Work out the finished part from the listing and answer in its coordinate system (mm). A direction names the side the tool comes from. Coordinates: 2 decimals unless noted, no trailing zeros. Order: outer loops, then holes, each group sorted by start corner. A loop starts at its lowest first (then second) coordinate and runs counter-clockwise, first axis right, second up. Notation, with made-up numbers: (-15, 12) -> (34, 12) arc R25 cw to (34, 48) -> close; hole circle Ø9 at (-22, 80). An arc over 180 degrees is marked (long way). Answer as CSV lines item,"result". Start each with the question number.
Item 1: Each of these flat-tipped pins is pushed along its axis until it touches: pin 1 Ø6 at (x, y) = (22, -3.5) entering from -Z; pin 2 Ø9.5 at (x, y) = (-26, -29.5) entering from -Z; pin 3 Ø8 at (x, z) = (-22.5, -22.5) entering from +Y; pin 4 Ø21 at (y, z) = (19, 26) entering from -X. Where does it stop, or does it pass through?
Item 2: Section D-D (y = 8) is taken. Write down the section's boundary in (x, z).
Item 3: Section A-A (z = 19.05) is taken. Write down the section's boundary in (x, y) (3 decimals).
Item 4: Section C-C (z = 2) is taken. Write down the section's boundary in (x, y).
Item 5: Straight lines are drawn through the part: L1, parallel to X at y = 1.85, z = 10; L2, parallel to Z at x = 5, y = 2; L3, parallel to Y at x = 34.8, z = -19.05 (3 decimals). For each, find the intervals that lie inside material, in ascending order.
Item 6: Which of the six approach directions +Z, -Z, +X, -X, +Y, -Y give full straight-line access (tool end or side, diameter ignored) to faces 1 (the face through (-5, 15, 27)), 2 (the face through (0, 15, -27)), 3 (the face through (-26, -15, -6.35))?
Item 7: Section B-B (x = 28.1) is taken. Write down the section's boundary in (y, z).
Item 8: For a pull along Y with two mould halves and no side action, classify faces 4 (the face through (5.03, 2.46, 11.5)), 5 (the face through (-29.69, -32.47, 0.09)), 6 (the face through (-2.46, 14.39, 12.36)) as pulls with the +Y half, pulls with the -Y half, needs draft (parallel to the pull), parting line crosses it, or undercut.
```python
from build123d import *

# Parameters (mm, degrees)
SKETCH2_W           = 76.2
SKETCH2_H           = 76.2
SKETCH2_R           = 1.5
BOSS_EXTRUDE1_DEPTH = 5
SKETCH3_W           = 76.2
SKETCH3_H           = 24.05
SKETCH3_R           = 4
BOSS_EXTRUDE2_DEPTH = 5
LPATTERN1_COUNT     = 2
LPATTERN1_PITCH     = 38.1
BOSS_EXTRUDE5_START = -38.1
SKETCH4_R           = 3
BOSS_EXTRUDE5_DEPTH = 6.35
CUT_EXTRUDE1_DEPTH  = 10


with BuildPart() as part:
    # Sketch2 → Boss-Extrude1 (new body)
    with BuildSketch(Plane(origin=(0, 0, 0), x_dir=(1, 0, 0), z_dir=(0, 1, 0))):
        Rectangle(SKETCH2_W, SKETCH2_H)
        with Locations(Location((28.1, 10, 0), (0, 0, 270))):
            Circle(SKETCH2_R, mode=Mode.SUBTRACT)
        with Locations(Location((5.1, 10, 0), (0, 0, 270))):
            Circle(SKETCH2_R, mode=Mode.SUBTRACT)
        with Locations(Location((28.1, -10, 0), (0, 0, 90))):
            Circle(SKETCH2_R, mode=Mode.SUBTRACT)
        with Locations(Location((5.1, -10, 0), (0, 0, 90))):
            Circle(SKETCH2_R, mode=Mode.SUBTRACT)
    extrude(amount=BOSS_EXTRUDE1_DEPTH)

    # Sketch3 → Boss-Extrude2 (add)
    with BuildSketch(Plane(origin=(38.1, 0, 0), x_dir=(0, 0, -1), z_dir=(1, 0, 0))):
        with Locations((0, 12.025)):
            Rectangle(SKETCH3_W, SKETCH3_H)
        with Locations((-19.05, 14.525)):
            Circle(SKETCH3_R, mode=Mode.SUBTRACT)
        with Locations((19.05, 14.525)):
            Circle(SKETCH3_R, mode=Mode.SUBTRACT)
    boss_extrude2 = extrude(amount=-BOSS_EXTRUDE2_DEPTH)

    # LPattern1: Boss-Extrude2 ×2
    with Locations(*[(-i * LPATTERN1_PITCH, 0, 0) for i in range(1, LPATTERN1_COUNT)]):
        add(boss_extrude2)

    # Sketch4 → Boss-Extrude5 (add, symmetric)
    with BuildSketch(Plane(origin=(0, 0, -38.1), x_dir=(-1, 0, 0), z_dir=(0, 0, -1)).offset(BOSS_EXTRUDE5_START)):
        with BuildLine():
            Line((6.1, 0), (38.1, 0))
            Line((38.1, 0), (38.1, -35.148267781))
            ThreePointArc((38.1, -35.148267781), (34.438424912, -39.965800215), (28.816552498, -37.72742995))
            Line((28.816552498, -37.72742995), (6.1, 0))
        make_face()
        with Locations((31.9, -34.5)):
            Circle(SKETCH4_R, mode=Mode.SUBTRACT)
    extrude(amount=BOSS_EXTRUDE5_DEPTH, both=True)

    # Sketch5 → Cut-Extrude1 (cut)
    with BuildSketch(Plane(origin=(0, 0, 0), x_dir=(0, 0, -1), z_dir=(1, 0, 0))):
        Polygon((9.743329583, 5), (-9.743329583, 5), (-15.05, 24.05), (-9.743329583, 24.05), (9.743329583, 24.05), (15.05, 24.05), align=None)
    extrude(amount=-CUT_EXTRUDE1_DEPTH, mode=Mode.SUBTRACT)


solid = part.part
```
Checked values:
1,pin 1,"passes through"
1,pin 2,"stops at z = -6.35"
1,pin 3,"stops at y = 5"
1,pin 4,"stops at x = -5"
2,outline,"(-5, -38.1) -> (0, -38.1) -> (0, -10.58) -> (-5, -10.58) -> close; (-5, 10.58) -> (0, 10.58) -> (0, 38.1) -> (-5, 38.1) -> close; (33.1, -38.1) -> (38.1, -38.1) -> (38.1, 38.1) -> (33.1, 38.1) -> close"
3,outline,"(-38.1, 0) -> (38.1, 0) -> (38.1, 10.525) -> (33.1, 10.525) -> (33.1, 5) -> (0, 5) -> (0, 10.525) -> (-5, 10.525) -> (-5, 5) -> (-38.1, 5) -> close; (-5, 18.525) -> (0, 18.525) -> (0, 24.05) -> (-5, 24.05) -> close; (33.1, 18.525) -> (38.1, 18.525) -> (38.1, 24.05) -> (33.1, 24.05) -> close"
4,outline,"(-38.1, -35.15) arc R5 ccw to (-28.82, -37.73) -> (-6.1, 0) -> (38.1, 0) -> (38.1, 24.05) -> (33.1, 24.05) -> (33.1, 5) -> (-38.1, 5) -> close; hole circle Ø6 at (-31.9, -34.5)"
5,L1,"x = -38.1 to 3.6, 6.6 to 26.6, 29.6 to 38.1"
5,L2,"z = -38.1 to -11.5, -8.5 to 8.5, 11.5 to 38.1"
5,L3,"y = 0 to 10.525, 18.525 to 24.05"
6,face 1,"+Z, -Z, -X, +Y"
6,face 2,"+Z, -Z, +Y"
6,face 3,"-Z, +X, -X, -Y"
7,outline,"(0, -38.1) -> (5, -38.1) -> (5, -11.5) -> (0, -11.5) -> close; (0, -8.5) -> (5, -8.5) -> (5, 8.5) -> (0, 8.5) -> close; (0, 11.5) -> (5, 11.5) -> (5, 38.1) -> (0, 38.1) -> close"
8,face 4,"needs draft"
8,face 5,"undercut"
8,face 6,"pulls with the +Y half"
